from build123d import *

# Parameters (mm, degrees)
F0_W     = 11
F0_H     = 4
F0_R     = 8.5
F1_DEPTH = 3
F2_DEPTH = 1
F0_W_2   = 3
F0_H_2   = 23
F0_H_3   = 3
F3_DEPTH = 14
F4_DEPTH = 10


with BuildPart() as f1:
    # F0 (on Front) → F1 (new body)
    with BuildSketch(Plane.XZ):
        Polygon((-5.5, 11.5), (-23.5, 11.5), (-23.5, -11.5), (-5.5, -11.5), (5.5, -11.5), (23.5, -11.5), (23.5, 11.5), (5.5, 11.5), align=None)
        with Locations((0, -8.5)):
            Rectangle(F0_W, F0_H, mode=Mode.SUBTRACT)
        with Locations((-13.5, 0)):
            Circle(F0_R, mode=Mode.SUBTRACT)
        with Locations((13.5, 0)):
            Circle(F0_R, mode=Mode.SUBTRACT)
    extrude(amount=F1_DEPTH)

    # F0 (on Front) → F2 (join)
    with BuildSketch(Plane.XZ):
        with Locations((0, -8.5)):
            Rectangle(F0_W, F0_H)
    extrude(amount=F2_DEPTH)

    # F0 (on Front) → F3 (join)
    with BuildSketch(Plane.XZ):
        Polygon((-26.5, 11.5), (-23.5, 11.5), (-5.5, 11.5), (-5.5, 14.5), (-26.5, 14.5), align=None)
        Polygon((5.5, 14.5), (5.5, 11.5), (23.5, 11.5), (26.5, 11.5), (26.5, 14.5), align=None)
        with Locations((-25, 0)):
            Rectangle(F0_W_2, F0_H_2)
        Polygon((23.5, -11.5), (5.5, -11.5), (5.5, -14.5), (26.5, -14.5), (26.5, -11.5), align=None)
        Polygon((-5.5, -11.5), (-23.5, -11.5), (-26.5, -11.5), (-26.5, -14.5), (-5.5, -14.5), align=None)
        with Locations((25, 0)):
            Rectangle(F0_W_2, F0_H_2)
        with Locations((0, -13)):
            Rectangle(F0_W, F0_H_3)
    extrude(amount=F3_DEPTH)

    # F0 (on Front) → F4 (join)
    with BuildSketch(Plane.XZ):
        with Locations((0, 13)):
            Rectangle(F0_W, F0_H_3)
    extrude(amount=F4_DEPTH)


solid = f1.part
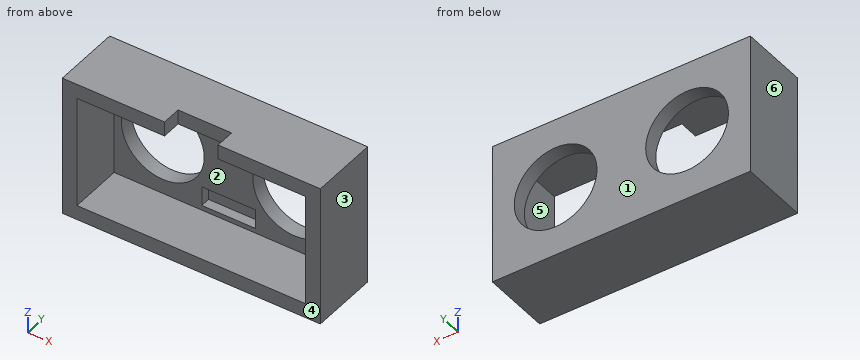
Geometry check sheet. Reference: the model listing, model coordinates, mm. Face numbers are marked on the shaded views. A direction names the side the tool comes from. Give positions to 0.01 mm unless a question says otherwise; leave off trailing zeros. Order: outer loops, then holes, each group sorted by start corner. A loop starts at its lowest first (then second) coordinate and runs counter-clockwise, first axis right, second up.
1) Cross-section at A-A (z = -7.5). Record the boundary of the cut face in (x, y).
Results are:
outline: (-26.5, -14) - (-23.5, -14) - (-23.5, -3) - (-17.5, -3) - (-17.5, 0) - (-26.5, 0) - close; (-9.5, -3) - (-5.5, -3) - (-5.5, -1) - (5.5, -1) - (5.5, -3) - (9.5, -3) - (9.5, 0) - (-9.5, 0) - close; (17.5, -3) - (23.5, -3) - (23.5, -14) - (26.5, -14) - (26.5, 0) - (17.5, 0) - close
2) Cross-section at B-B (x = 13.5). Record the boundary of the cut face in (y, z).
Results are:
outline: (-14, -14.5) - (0, -14.5) - (0, -8.5) - (-3, -8.5) - (-3, -11.5) - (-14, -11.5) - close; (-14, 11.5) - (-3, 11.5) - (-3, 8.5) - (0, 8.5) - (0, 14.5) - (-14, 14.5) - close
3) Cross-section at D-D (y = -13). Record the boundary of the cut face in (x, z).
Results are:
outline: (-26.5, -14.5) - (26.5, -14.5) - (26.5, 14.5) - (5.5, 14.5) - (5.5, 11.5) - (23.5, 11.5) - (23.5, -11.5) - (-23.5, -11.5) - (-23.5, 11.5) - (-5.5, 11.5) - (-5.5, 14.5) - (-26.5, 14.5) - close
4) Draft check along X on the marked faces 3, 4, 5 and 6. Enter one of: released by +X, released by -X, zero draft, split by the parting line, or undercut.
Results are:
face 3: released by +X
face 4: zero draft
face 5: undercut
face 6: released by -X
5) Tool access check on the marked faces 1 and 2. Record the directions out of +Z, -Z, +X, -X, +Y, -Y that give a thin tool (end or side, any length) a straight path to the whole face; none if there is none.
Results are:
face 1: +Z, -Z, +X, -X, +Y
face 2: -Y
6) Material ranges on probe 1 along Z at (x, y) = (-19, -9.5); probe 2 along X at (y, z) = (-7.75, -10.25); probe 3 along Z at (x, y) = (-13.5, -0.65), recorded low to high.
Results are:
probe 1: z = -14.5 to -11.5, 11.5 to 14.5
probe 2: x = -26.5 to -23.5, 23.5 to 26.5
probe 3: z = -14.5 to -8.5, 8.5 to 14.5
7) Gauge pin test, flat ends, axial feed: pin 1 (1.5 mm diameter, centred on x = -2, z = 13.5, fed in from -Y); pin 2 (5 mm diameter, centred on x = -6.5, z = -5.5, fed in from -Y); pin 3 (2 mm diameter, centred on x = 1.5, z = -8, fed in from -Y). Record the tip position at first contact, or that the pin passes through.
Results are:
pin 1: stops at y = -10
pin 2: stops at y = -3
pin 3: stops at y = -1
8) Cross-section at C-C (y = -3.75). Record the boundary of the cut face in (x, z), then the cut area to 3 significant figures.
Results are:
outline: (-26.5, -14.5) - (26.5, -14.5) - (26.5, 14.5) - (-26.5, 14.5) - close; hole (-23.5, -11.5) - (23.5, -11.5) - (23.5, 11.5) - (-23.5, 11.5) - close
area: 456 mm2
